The model under review builds one solid part; all positions refer to its coordinate system, in mm. A direction names the side the tool comes from. Round coordinates to 2 decimals unless told otherwise and drop trailing zeros. Write each loop counter-clockwise with the first axis right and the second up, starting at its lowest first coordinate (ties: lowest second). Pieces come first, ordered by that corner, then holes.
Item 1: To check wall thickness, follow L1, parallel to Y at x = -3, z = 0.55; L2, parallel to Y at x = -28.5, z = 25; L3, parallel to X at y = 14, z = 16.5. State the ranges of each line that lie inside material, in increasing order.
Item 2: Add section B-B (x = -3). Give the boundary of the cut face in (y, z).
Item 3: Add section A-A (z = 25). Give the boundary of the cut face in (x, y).
Item 4: Machinability: for faces 1 (the face through (0, 0, 1)), 2 (the face through (-28, 0, 16)), which of the approach directions +Z, -Z, +X, -X, +Y, -Y give a long, thin tool a straight path to every point of the face, cutting with its end or side? Answer none if there is none.
Item 5: Clearance check with flat-ended pins moving along their axes: pin 1 Ø3 at (x, y) = (-3, 15.5) entering from -Z (1 decimal); pin 2 Ø4 at (y, z) = (0, 25) entering from +X; pin 3 Ø10 at (x, z) = (-24, 13.5) entering from -Y; pin 4 Ø8.5 at (x, y) = (-15, 4.5) entering from +Z. State where each tip first meets the part, or that it passes through.
Item 6: Add section C-C (y = -10.5). Give the boundary of the cut face in (x, z), plus the area to 3 significant figures.
Item 7: Add section D-D (y = 15.5). Give the boundary of the cut face in (x, z), plus the area to 3 significant figures.
Item 8: Draft analysis for pull direction Z (two halves, no side actions). For faces 3 (the face through (-15, 0, 0)), 4 (the face through (-3.234, 17.285, 0.986)), 5 (the face through (-28.986, -0.594, 23.568)), state which applies: +Z half, -Z half, draft (parallel to the pull), parting line (faces both ways), or undercut.
```python
from build123d import *

# Parameters (mm, degrees)
SKETCH1_W           = 30
SKETCH1_H           = 41
SKETCH1_R           = 1.8
BOSS_EXTRUDE1_DEPTH = 2
SKETCH2_W           = 2
SKETCH2_H           = 41
BOSS_EXTRUDE2_DEPTH = 28
SKETCH3_R           = 1.55
CUT_EXTRUDE1_DEPTH  = 10


with BuildPart() as part:
    # Sketch1 → Boss-Extrude1 (new body)
    with BuildSketch(Plane.XY):
        with Locations((-15, 0)):
            Rectangle(SKETCH1_W, SKETCH1_H)
        with Locations((-3, 15.5)):
            Circle(SKETCH1_R, mode=Mode.SUBTRACT)
        with Locations((-3, -15.5)):
            Circle(SKETCH1_R, mode=Mode.SUBTRACT)
    extrude(amount=BOSS_EXTRUDE1_DEPTH)

    # Sketch2 → Boss-Extrude2 (add)
    with BuildSketch(Plane.XY.offset(2)):
        with Locations((-29, 0)):
            Rectangle(SKETCH2_W, SKETCH2_H)
    extrude(amount=BOSS_EXTRUDE2_DEPTH)

    # Sketch3 → Cut-Extrude1 (cut)
    with BuildSketch(Plane(origin=(-28, 0, 0), x_dir=(0, 0, -1), z_dir=(1, 0, 0))):
        with Locations((-25, 10.5)):
            Circle(SKETCH3_R)
        with Locations((-25, -10.5)):
            Circle(SKETCH3_R)
        with Locations((-25, 0)):
            Circle(SKETCH3_R)
        Polygon((-30, -13.5), (-23, -20.5), (-30, -20.5), align=None)
        Polygon((-30, 13.5), (-30, 20.5), (-23, 20.5), align=None)
    extrude(amount=-CUT_EXTRUDE1_DEPTH, mode=Mode.SUBTRACT)


solid = part.part
```
Numbers:
1. L1: y = -20.5 to -17.3, -13.7 to 13.7, 17.3 to 20.5
1. L2: y = -18.5 to -12.05, -8.95 to -1.55, 1.55 to 8.95, 12.05 to 18.5
1. L3: x = -30 to -28
2. outline: (-20.5, 0) - (-17.3, 0) - (-17.3, 2) - (-20.5, 2) - close; (-13.7, 0) - (13.7, 0) - (13.7, 2) - (-13.7, 2) - close; (17.3, 0) - (20.5, 0) - (20.5, 2) - (17.3, 2) - close
3. outline: (-30, -18.5) - (-28, -18.5) - (-28, -12.05) - (-30, -12.05) - close; (-30, -8.95) - (-28, -8.95) - (-28, -1.55) - (-30, -1.55) - close; (-30, 1.55) - (-28, 1.55) - (-28, 8.95) - (-30, 8.95) - close; (-30, 12.05) - (-28, 12.05) - (-28, 18.5) - (-30, 18.5) - close
4. face 1: +Z, -Z, +X, +Y, -Y
4. face 2: +Z, +X, +Y, -Y
5. pin 1: passes through
5. pin 2: stops at x = -28
5. pin 3: stops at y = -20.5
5. pin 4: stops at z = 2
6. outline: (-30, 0) - (0, 0) - (0, 2) - (-28, 2) - (-28, 23.45) - (-30, 23.45) - close; (-30, 26.55) - (-28, 26.55) - (-28, 30) - (-30, 30) - close
6. area: 110 mm2
7. outline: (-30, 0) - (-4.8, 0) - (-4.8, 2) - (-28, 2) - (-28, 28) - (-30, 28) - close; (-1.2, 0) - (0, 0) - (0, 2) - (-1.2, 2) - close
7. area: 105 mm2
8. face 3: -Z half
8. face 4: draft
8. face 5: undercut
